Source: CAD feature listing. Evaluate the final solid. Frame: model axes, mm. Face numbers are marked on the shaded views. A direction names the side the tool comes from. Give positions to 0.01 mm unless a question says otherwise; leave off trailing zeros. Write each loop counter-clockwise with the first axis right and the second up, starting at its lowest first coordinate (ties: lowest second). Pieces come first, ordered by that corner, then holes. Notation, with made-up numbers: (55.25, -26.75) - (84.25, -26.75) arc R29 cw to (84.25, 4.25) - close; hole circle Ø7 at (14.25, -12.5). An arc over 180 degrees is marked (long way). Answer as a JSON object with one key per item and string values. Group by question number.
from build123d import *

# Parameters (mm, degrees)
SKIZZE1_W                       = 61.8
SKIZZE1_H                       = 93.64
AUFSATZ_LINEAR_AUSTRAGEN1_DEPTH = 10
VERRUNDUNG1_R                   = 6
WANDUNG1_T                      = -1
SKIZZE2_W                       = 21.5
SKIZZE2_H                       = 15.5
SCHNITT_LINEAR_AUSTRAGEN1_DEPTH = 6
SKIZZE3_W                       = 22
SKIZZE3_H                       = 8
SCHNITT_LINEAR_AUSTRAGEN2_DEPTH = 6
SCHNITT_LINEAR_AUSTRAGEN4_DEPTH = 6
LINEARES_MUSTER1_COUNT          = 3
LINEARES_MUSTER1_PITCH          = 25


with BuildPart() as part:
    # Skizze1 → Aufsatz-Linear austragen1 (new body)
    with BuildSketch(Plane(origin=(0, 0, 0), x_dir=(0, 1, 0), z_dir=(0, 0, 1))):
        Rectangle(SKIZZE1_W, SKIZZE1_H)
    extrude(amount=AUFSATZ_LINEAR_AUSTRAGEN1_DEPTH)

    # Verrundung1
    verrundung1_edges = [part.edges().sort_by_distance(p)[0] for p in [
        (46.82, 30.9, 5),
        (46.82, -30.9, 5),
        (-46.82, -30.9, 5),
        (-46.82, 30.9, 5),
    ]]
    fillet(verrundung1_edges, radius=VERRUNDUNG1_R)

    # Wandung1
    wandung1_openings = [part.faces().sort_by_distance(p)[0] for p in [
        (0, 0, 10),
    ]]
    offset(amount=WANDUNG1_T, openings=wandung1_openings, kind=Kind.INTERSECTION)

    # Skizze2 → Schnitt-Linear austragen1 (cut)
    with BuildSketch(Plane.YZ.offset(46.82)):
        with Locations((0, 10)):
            Rectangle(SKIZZE2_W, SKIZZE2_H)
    extrude(amount=-SCHNITT_LINEAR_AUSTRAGEN1_DEPTH, mode=Mode.SUBTRACT)

    # Skizze3 → Schnitt-Linear austragen2 (cut)
    with BuildSketch(Plane.XZ.offset(30.9)):
        with Locations((-9.18, 6)):
            Rectangle(SKIZZE3_W, SKIZZE3_H)
    extrude(amount=-SCHNITT_LINEAR_AUSTRAGEN2_DEPTH, mode=Mode.SUBTRACT)

    # Skizze4 → Schnitt-Linear austragen4 (cut)
    with BuildSketch(Plane(origin=(0, 0, 0), x_dir=(1, 0, 0), z_dir=(0, 0, -1))):
        Polygon((-18.82, -2.339745962), (-28.82, -2.339745962), (-33.82, -11), (-28.82, -19.660254038), (-18.82, -19.660254038), (-13.82, -11), align=None)
    schnitt_linear_austragen4 = extrude(amount=-SCHNITT_LINEAR_AUSTRAGEN4_DEPTH, mode=Mode.SUBTRACT)

    # Lineares Muster1: Schnitt-Linear austragen4 ×3
    with Locations(*[(i * LINEARES_MUSTER1_PITCH, 0, 0) for i in range(1, LINEARES_MUSTER1_COUNT)]):
        add(schnitt_linear_austragen4, mode=Mode.SUBTRACT)


solid = part.part
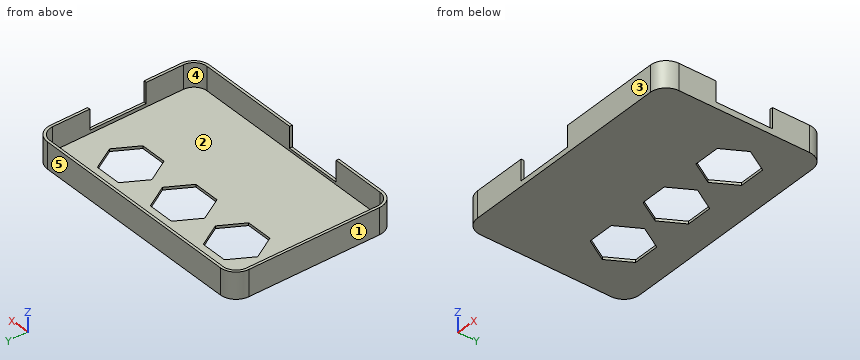
Q1. Ray query, probe 1 along Y at (x, z) = (10, 7); probe 2 along X at (y, z) = (23.5, 5); probe 3 along Z at (x, y) = (23, 22.5). Return the intervals inside material, ascending. Write a range as [from, to].
Q2. Section B-B on x = -31.5. Return the cut outline in (y, z), then the cut area to 3 significant figures.
Q3. Draft query along Y for the marked faces 1, 2 and 3. Return one class per face: released by +Y, released by -Y, zero draft, split by the parting line, or undercut.
Q4. Section D-D on y = -17.5. Return the cut outline in (x, z), then the cut area to 3 significant figures.
Q5. Reachability of the marked faces 4 and 5 from +Z, -Z, +X, -X, +Y, -Y: full face, straight path, thin tool, end or side. Return the list, or none.
Q6. First-contact query: pin 1 Ø0.8 at (x, y) = (46, -0.5) entering from +Z; pin 2 Ø0.5 at (y, z) = (-30.5, 5) entering from -X; pin 3 Ø1 at (x, y) = (-8.5, 11.5) entering from +Z. Flat tips, straight axial feed; report the tip coordinate or a pass-through.
Q7. Section A-A on z = 4. Return the cut outline in (x, y).
Q8. Section C-C on y = 4. Return the cut outline in (x, z).
Taken from the geometry:
{
 "1": {"probe 1": "y = [-30.9, -29.9], [29.9, 30.9]", "probe 2": "x = [-46.82, -45.82], [45.82, 46.82]", "probe 3": "z = [0, 1]"},
 "2": {"outline": "(-30.9, 0) - (6.98, 0) - (6.98, 1) - (-29.9, 1) - (-29.9, 10) - (-30.9, 10) - close; (15.02, 0) - (30.9, 0) - (30.9, 10) - (29.9, 10) - (29.9, 1) - (15.02, 1) - close", "area": "71.8 mm²"},
 "3": {"face 1": "zero draft", "face 2": "undercut", "face 3": "released by -Y"},
 "4": {"outline": "(-46.82, 0) - (46.82, 0) - (46.82, 10) - (45.82, 10) - (45.82, 1) - (-45.82, 1) - (-45.82, 10) - (-46.82, 10) - close", "area": "112 mm²"},
 "5": {"face 4": "+Z", "face 5": "+Z, -Z, +X, -X, +Y"},
 "6": {"pin 1": "stops at z = 2.25", "pin 2": "stops at x = -43.54", "pin 3": "stops at z = 1"},
 "7": {"outline": "(-46.82, -24.9) arc R6 ccw to (-40.82, -30.9) - (-20.18, -30.9) - (-20.18, -29.9) - (-40.82, -29.9) arc R5 cw to (-45.82, -24.9) - (-45.82, 24.9) arc R5 cw to (-40.82, 29.9) - (40.82, 29.9) arc R5 cw to (45.82, 24.9) - (45.82, 10.75) - (46.82, 10.75) - (46.82, 24.9) arc R6 ccw to (40.82, 30.9) - (-40.82, 30.9) arc R6 ccw to (-46.82, 24.9) - close; (1.82, -30.9) - (40.82, -30.9) arc R6 ccw to (46.82, -24.9) - (46.82, -10.75) - (45.82, -10.75) - (45.82, -24.9) arc R5 cw to (40.82, -29.9) - (1.82, -29.9) - close"},
 "8": {"outline": "(-46.82, 0) - (-29.78, 0) - (-29.78, 1) - (-45.82, 1) - (-45.82, 10) - (-46.82, 10) - close; (-17.86, 0) - (-4.78, 0) - (-4.78, 1) - (-17.86, 1) - close; (7.14, 0) - (20.22, 0) - (20.22, 1) - (7.14, 1) - close; (32.14, 0) - (46.82, 0) - (46.82, 2.25) - (45.82, 2.25) - (45.82, 1) - (32.14, 1) - close"}
}
